Autodesk Inventor part; units mm, degrees
ref_plane "YZ Plane" through (0, 0, 0) normal (1, 0, 0) x (0, 1, 0)
ref_plane "XZ Plane" through (0, 0, 0) normal (0, 1, 0) x (-1, 0, 0)
ref_plane "XY Plane" through (0, 0, 0) normal (0, 0, 1) x (1, 0, 0)
sketch "Sketch1" plane through (0, 0, 0) normal (0, 1, 0) x (-1, 0, 0)
  line L0 (0, 0) -> (-228.6, 0)
  line L1 (-228.6, 0) -> (-228.6, -82.55)
  line L2 (0, 0) -> (0, -82.55)
  line L3 (-228.6, 0) -> (-222.25, 0)
  circle A0 centre (-222.25, -6.35) radius 2.3241
  circle A1 centre (-222.25, -31.75) radius 2.3241
  line L4 (-228.6, 0) -> (-114.3, 0)
  line L5 (-114.3, 0) -> (-114.3, 9.4502)
  circle A2 centre (-222.25, -69.85) radius 2.3241
  circle A3 centre (-6.35, -6.35) radius 2.3241
  circle A4 centre (-6.35, -31.75) radius 2.3241
  circle A5 centre (-6.35, -69.85) radius 2.3241
  line L6 (-228.6, -82.55) -> (-215.9, -82.55)
  line L7 (0, -82.55) -> (-12.7, -82.55)
  line L8 (-114.3, 0) -> (-114.3, -38.1)
  arc A6 (-12.7, -82.55) -> (-215.9, -82.55) centre (-114.3, -176.4393) ccw
  line L9 (-228.6, 0) -> (-231.775, 0)
  line L10 (-231.775, 0) -> (-231.775, -82.55)
  line L11 (-231.775, -82.55) -> (-228.6, -82.55)
  line L12 (-228.6, 0) -> (-228.6, 3.175)
  line L13 (-228.6, 3.175) -> (-231.775, 3.175)
  line L14 (-231.775, 3.175) -> (-231.775, 0)
  line L15 (-228.6, 3.175) -> (0, 3.175)
  line L16 (0, 3.175) -> (0, 0)
  line L17 (0, 0) -> (3.175, 0)
  line L18 (3.175, 0) -> (3.175, 3.175)
  line L19 (3.175, 3.175) -> (0, 3.175)
  line L20 (3.175, 0) -> (3.175, -82.55)
  line L21 (3.175, -82.55) -> (0, -82.55)
  point P0 (-225.425, 0)
  dimension "d0" = 228.6
  dimension "d1" = 82.55
  dimension "d2" = 6.35
  dimension "d4" = 4.6482
  dimension "d6" = 4.6482
  dimension "d7" = 114.3
  dimension "d9" = 4.6482
  dimension "d10" = 6.35
  dimension "d11" = 31.75
  dimension "d12" = 69.85
  dimension "d14" = 12.7
  dimension "d15" = 12.7
  dimension "d16" = 38.1
  dimension "d20" = 3.175
  dimension "d21" = 3.175
  dimension "d22" = 3.175
extrude "Extrusion1" add sketch "Sketch1" against normal blind 3.175 contours L2 L7 A6 L8 L0 | L8 A6 L6 L1 L0
fillet "Fillet1" radius 8.4667 4 edges at (228.6, -1.5875, -82.55) (215.9, -1.5875, -82.55) (12.7, -1.5875, -82.55) (0, -1.5875, -82.55)
extrude "Extrusion2" add sketch "Sketch1" against normal blind 6.35
fillet "Fillet2" radius 8.4667 4 edges at (231.775, -3.175, -82.55) (231.775, -3.175, 3.175) (-3.175, -3.175, 3.175) (-3.175, -3.175, -82.55)
fillet "Fillet3" radius 12.7 2 edges at (215.9, -3.175, -82.55) (12.7, -3.175, -82.55)
properties part number "Intake (Plastic)"
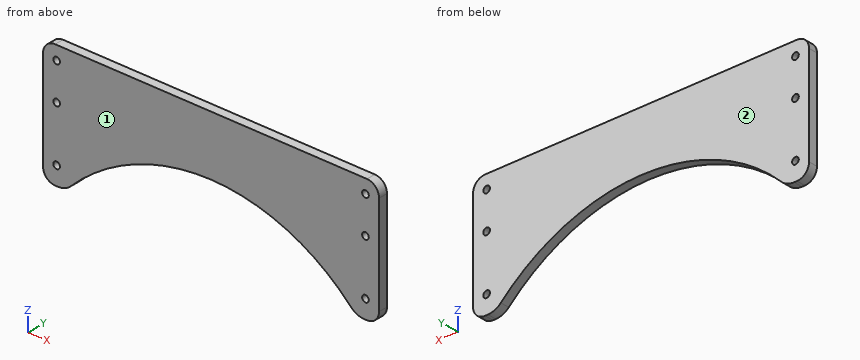
The listing builds one solid part. Answer for the finished solid, in the listing's coordinates (mm). Face numbers are marked on the shaded views. Coordinates: 2 decimals unless noted, no trailing zeros. Loops run counter-clockwise (first coordinate to the right, second up) from the corner with the lowest first, then second, coordinate; pieces in that order, holes last. Notation, with made-up numbers: M 60,27 L 83,27 A17 ccw 83,53 Z; hole C 33,70.25 d8. An arc over 180 degrees is marked long. Answer as a JSON object with one key per item and string values. Group by question number.
Item 1: Section B-B (y = -4.75) is taken. Write down the section's boundary in (x, z) (3 decimals), and give its area (3 significant figures).
Item 2: Determine the mould class of the marked faces 1 and 2 for opening direction Y: +Y half, -Y half, draft (parallel to the pull), parting line (faces both ways), or undercut.
Item 3: Section C-C (z = -55.5) is taken. Write down the section's boundary in (x, y) (3 decimals), and give its area (3 significant figures).
Item 4: Section A-A (z = -31.75) is taken. Write down the section's boundary in (x, y) (3 decimals).
Item 5: Section D-D (z = -69.85) is taken. Write down the section's boundary in (x, y) (3 decimals).
Item 6: Consider L1, parallel to Z at x = 6.35, y = -4.5 (3 decimals); L2, parallel to X at y = -1.75, z = -30 (3 decimals); L3, parallel to X at y = -4.5, z = -7.5 (3 decimals). Determine where each line is inside the solid, lowest interval first.
Solved:
{
 "1": {"outline": "M -3.175,-74.083 A8.467 ccw 5.292,-82.55 L 7.288,-82.55 A12.7 ccw 16.286,-78.812 A138.339 cw 212.314,-78.812 A12.7 ccw 221.312,-82.55 L 223.308,-82.55 A8.467 ccw 231.775,-74.083 L 231.775,-5.292 A8.467 ccw 223.308,3.175 L 5.292,3.175 A8.467 ccw -3.175,-5.292 Z; hole C 6.35,-69.85 d4.648; hole C 6.35,-31.75 d4.648; hole C 6.35,-6.35 d4.648; hole C 222.25,-69.85 d4.648; hole C 222.25,-31.75 d4.648; hole C 222.25,-6.35 d4.648", "area": "13,700 mm2"},
 "2": {"face 1": "-Y half", "face 2": "+Y half"},
 "3": {"outline": "M -3.175,-6.35 L 47.133,-6.35 L 47.133,0 L -3.175,0 Z; M 181.467,-6.35 L 231.775,-6.35 L 231.775,0 L 181.467,0 Z", "area": "639 mm2"},
 "4": {"outline": "M -3.175,-6.35 L 4.026,-6.35 L 4.026,0 L -3.175,0 Z; M 8.674,-6.35 L 219.926,-6.35 L 219.926,0 L 8.674,0 Z; M 224.574,-6.35 L 231.775,-6.35 L 231.775,0 L 224.574,0 Z"},
 "5": {"outline": "M -3.175,-6.35 L 4.026,-6.35 L 4.026,0 L -3.175,0 Z; M 8.674,-6.35 L 26.116,-6.35 L 26.116,0 L 8.674,0 Z; M 202.484,-6.35 L 219.926,-6.35 L 219.926,0 L 202.484,0 Z; M 224.574,-6.35 L 231.775,-6.35 L 231.775,0 L 224.574,0 Z"},
 "6": {"L1": "z = -82.55 to -72.174, -67.526 to -34.074, -29.426 to -8.674, -4.026 to 3.175", "L2": "x = -3.175 to 4.821, 7.879 to 220.721, 223.779 to 231.775", "L3": "x = -3.175 to 4.33, 8.37 to 220.23, 224.27 to 231.775"}
}
